Could you check a few things on this model? Use its own coordinates, in mm. A direction names the side the tool comes from. Coordinates: 2 decimals unless noted, no trailing zeros. Loops run counter-clockwise (first coordinate to the right, second up) from the corner with the lowest first, then second, coordinate; pieces in that order, holes last. Notation, with made-up numbers: M -22,-37.75 L 13,-37.75 A29 cw 13,1.25 Z; hole C 89.25,-32.75 d3. An arc over 180 degrees is marked long. Write each question's results on one line, items separated by ' | '.
Autodesk Inventor part; units mm, degrees
ref_plane "Work Plane1" through (29.8423, 0, 0) normal (0, 0, 1) x (-1, 0, 0)
ref_plane "YZ Plane" through (0, 0, 0) normal (1, 0, 0) x (0, 1, 0)
ref_plane "XZ Plane" through (0, 0, 0) normal (0, 1, 0) x (-1, 0, 0)
sketch "Náčrt1" plane through (0, 0, 0) normal (1, 0, 0) x (0, 1, 0)
  line L0 (-10.3923, 0) -> (-5.1962, 9)
  line L1 (-5.1962, 9) -> (5.1962, 9)
  line L2 (5.1962, 9) -> (10.3923, 0)
  line L3 (10.3923, 0) -> (5.1962, -9)
  line L4 (5.1962, -9) -> (-5.1962, -9)
  line L5 (-5.1962, -9) -> (-10.3923, 0)
  point P0 (0, 0)
  point P1 (0, 0)
  dimension "d0" = 20.7846
extrude "Těleso" add sketch "Náčrt1" along normal blind 11.6
sketch "Náčrt2" plane through (0, 0, 0) normal (-1, 0, 0) x (0, 0, 1)
  line L0 (0, -14.5492) -> (0, 14.5492)
  line L1 (-12.6, 0) -> (12.6, 0)
  point P0 (0, 0)
hole "Závit" at (0, 0, 0) direction (1, 0, 0) diameter 10.106 end through all
chamfer "Zkosení1" distance 0.9472 angle 30 1 edges at (0, 0, -5.053) measured on face at (0, -6.5823, -3.9568)
chamfer "Zkosení2" distance 0.9472 angle 30 1 edges at (11.6, 0, -5.053) measured on face at (11.6, -6.5823, -3.9568)
sketch "Náčrt3" plane through (0, 0, 0) normal (0, 0, 1) x (1, 0, 0)
  line L0 (0, 5.1962) -> (0, 10.3923)
  line L1 (0, 10.3923) -> (11.6, 10.3923)
  line L2 (11.6, 5.1962) -> (11.6, 10.3923)
  line L3 (-2.32, 0) -> (13.92, 0)
  line L4 (0.8038, 10.3923) -> (0, 9)
  line L5 (11.6, 7.65) -> (9.9682, 7.65)
  line L6 (9.9682, 7.65) -> (6.7, 10.3923)
  dimension "d3" = 30
  dimension "d5" = 18
  dimension "d6" = 15.3
  dimension "d8" = 50
  dimension "d9" = 6.7
revolve "Zkosení3" cut sketch "Náčrt3" angle 360 about axis through (-10, 0, 0) along (1, 0, 0)
ref_plane "Work Plane1" through (29.8423, 0, 0) normal (0, 0, 1) x (-1, 0, 0)
equation "\"d0\" = 1.1547 * SW"
equation "\"d1\" = KOH"
equation "\"d3\" = ANG1"
equation "\"d5\" = SW0"
equation "\"d6\" = SW1"
equation "\"d8\" = ANG2"
equation "\"d9\" = KOH1"
equation "\"d10\" = -0.5 * GD1 + 0.5 * NND"
equation "\"d39\" = -0.5 * GD1 + 0.5 * NND"
equation "\"d12\" = -0.5 * GD1 + 0.5 * NND"
equation "\"d40\" = -0.5 * GD1 + 0.5 * NND"
equation "\"ANG1\" = 30deg"
equation "\"ANG2\" = 50deg"
equation "\"NND\" = 12"
equation "\"KOH\" = 11.6"
equation "\"SW\" = 18"
equation "\"SW0\" = SW"
equation "\"SW1\" = 0.85 * SW"
equation "\"KOH1\" = 6.7"
equation "\"GUL\" = 0.541266 * PTC"
equation "\"THREADDIA\" = 12"
equation "\"TOA\" = 30deg"
equation "\"PTC\" = 1.75"
equation "\"E0\" = 1.155 * SW"
equation "\"GAL\" = 0.541266 * PTC"
properties part number "ANSI B18.16.3M - Property Class 5 and 10 - Metric M12 x 1.75 Typ kovu" material "Ocel, měkká"
(1) Please list where these lines run through material, in increasing order: probe 1 along Z at (x, y) = (7, 0); probe 2 along Y at (x, z) = (7.5, 0); probe 3 along Y at (x, z) = (7.5, 1.75). Write a range as from..to.
Reported:
probe 1: z = -9..-5.05, 5.05..9 | probe 2: y = -9.72..-5.05, 5.05..9.72 | probe 3: y = -9.38..-4.74, 4.74..9.38
(2) Imagine slicing it at A-A, the plane x = 4. List the corners of the cut face in (y, z) for me.
Reported:
outline: M -10.39,0 L -5.2,-9 L 5.2,-9 L 10.39,0 L 5.2,9 L -5.2,9 Z; hole C 0,0 d10.11
(3) If we mould it in two halves opening along Y, with no side actions, what happens to faces 1 (the cylindrical face through (5.874, 3.075, -4.01)), 2 (the conical face through (0.195, 9.338, -0.023)), 3 (the conical face through (0.2, -4.69, -8.08))? For each: released by +Y, released by -Y, zero draft, split by the parting line, or undercut.
Reported:
face 1: undercut | face 2: released by +Y | face 3: released by -Y
(4) Will these pins go through, and if not, where does the flat tip stop? P1, Ø3, axis at x = 9, z = 5.5, coming from the -Y side; P2, Ø4, axis at x = 4, z = -5.5, coming from the -Y side; P3, Ø6, axis at y = 0, z = 0, coming from the -X side; P4, Ø1.5, axis at x = 2.5, z = 7, coming from the +Y side.
Reported:
P1: stops at y = -8 | P2: stops at y = -8.37 | P3: passes through | P4: stops at y = 6.78
(5) Which directions (+Z, -Z, +X, -X, +Y, -Y) give clear straight access to the entire face, cutting with the end or side of a thin tool? Please do faces 4 (the flat face through (4, 0, 9)), 5 (the cylindrical face through (10.773, -1.658, 7.468)).
Reported:
face 4: +Z, +X, -X, +Y, -Y | face 5: +X
